The listing builds one solid part. Answer for the finished solid, in the listing's coordinates (mm). A direction names the side the tool comes from. Coordinates: 2 decimals unless noted, no trailing zeros. Write each loop counter-clockwise with the first axis right and the second up, starting at its lowest first coordinate (ties: lowest second). Pieces come first, ordered by that corner, then holes. Notation, with made-up numbers: M -9.75,34 L 48.25,34 A9 cw 48.25,41 Z; hole C 31.25,53.25 d10. An arc over 180 degrees is marked long. Put each result on its own line as item: value. Start each with the question number.
```python
from build123d import *

# Parameters (mm, degrees)
SKETCH1_R               = 16.5
SKETCH1_R_2             = 12
BOSS_EXTRUDE1_DEPTH     = 81.5
BOSS_EXTRUDE2_START     = -5
SKETCH2_R               = 38
BOSS_EXTRUDE2_DEPTH     = 153
SKETCH3_R               = 12
CUT_EXTRUDE1_DEPTH      = 167.88918479
CUT_EXTRUDE1_DEPTH_BACK = 167.88918479


with BuildPart() as part:
    # Sketch1 → Boss-Extrude1 (new, symmetric)
    with BuildSketch(Plane(origin=(0, 0, 0), x_dir=(0, 0, -1), z_dir=(1, 0, 0))):
        Circle(SKETCH1_R)
        Circle(SKETCH1_R_2, mode=Mode.SUBTRACT)
    extrude(amount=BOSS_EXTRUDE1_DEPTH, both=True)

    # Sketch2 → Boss-Extrude2 (add)
    with BuildSketch(Plane.ZY.offset(81.5).offset(BOSS_EXTRUDE2_START)):
        Circle(SKETCH2_R)
    extrude(amount=-BOSS_EXTRUDE2_DEPTH)

    # Sketch3 → Cut-Extrude1 (cut, two sides)
    with BuildSketch(Plane.ZY.offset(76.5)) as cut_extrude1_sk:
        with Locations(Location((0, 0, 0), (0, 0, 180))):
            Circle(SKETCH3_R)
    extrude(amount=CUT_EXTRUDE1_DEPTH, mode=Mode.SUBTRACT)
    extrude(cut_extrude1_sk.sketch, amount=-CUT_EXTRUDE1_DEPTH_BACK, mode=Mode.SUBTRACT)


solid = part.part
```
1) Given pin 1 Ø1 at (x, y) = (60.5, 30) entering from +Z; pin 2 Ø6 at (y, z) = (11, -27) entering from -X; pin 3 Ø2 at (x, z) = (-16.5, 1.5) entering from -Y, each flat-ended and moving along its own axis, determine where each tip first touches the part or whether it passes through.
2) Straight lines are drawn through the part: probe 1 along Y at (x, z) = (79.4, 0); probe 2 along X at (y, z) = (-6.5, 28); probe 3 along Y at (x, z) = (50.5, 6.5). For each, find the intervals that lie inside material, in ascending order.
3) A cutting plane is placed at C-C on x = -26.5. Write down the section's boundary in (y, z), then the cut area to 3 significant figures.
4) A cutting plane is placed at A-A on y = 0. Write down the section's boundary in (x, z).
5) For faces 1 (the face through (79.04, -6.32, -15.24)), 2 (the face through (-81.5, -12.15, -1.15)), 3 (the face through (-78.96, -6.32, -15.24)), determine the directions among +Z, -Z, +X, -X, +Y, -Y from which every point of the face is accessible in a straight line to the end or side of a thin tool.
6) A cutting plane is placed at B-B on z = 4. Write down the section's boundary in (x, y).
7) A cutting plane is placed at D-D on y = -31.5. Write down the section's boundary in (x, z), then the cut area to 3 significant figures.
Answers follow:
1. pin 1: stops at z = 23.95
1. pin 2: stops at x = -76.5
1. pin 3: stops at y = -38
2. probe 1: y = -16.5 to -12, 12 to 16.5
2. probe 2: x = -76.5 to 76.5
2. probe 3: y = -37.44 to -10.09, 10.09 to 37.44
3. outline: C 0,0 d76; hole C 0,0 d24
3. area: 4,080 mm²
4. outline: M -81.5,-16.5 L -76.5,-16.5 L -76.5,-38 L 76.5,-38 L 76.5,-16.5 L 81.5,-16.5 L 81.5,-12 L -81.5,-12 Z; M -81.5,12 L 81.5,12 L 81.5,16.5 L 76.5,16.5 L 76.5,38 L -76.5,38 L -76.5,16.5 L -81.5,16.5 Z
5. face 1: +X
5. face 2: +Z, -Z, -X, +Y, -Y
5. face 3: -X
6. outline: M -81.5,-16.01 L -76.5,-16.01 L -76.5,-37.79 L 76.5,-37.79 L 76.5,-16.01 L 81.5,-16.01 L 81.5,-11.31 L -81.5,-11.31 Z; M -81.5,11.31 L 81.5,11.31 L 81.5,16.01 L 76.5,16.01 L 76.5,37.79 L -76.5,37.79 L -76.5,16.01 L -81.5,16.01 Z
7. outline: M -76.5,-21.25 L 76.5,-21.25 L 76.5,21.25 L -76.5,21.25 Z
7. area: 6,500 mm²
